Could you check a few things on this model? Use its own coordinates, in mm. A direction names the side the tool comes from. Round coordinates to 2 decimals unless told otherwise and drop trailing zeros. Write each loop counter-clockwise with the first axis right and the second up, starting at its lowest first coordinate (ties: lowest second). Pieces come first, ordered by that corner, then holes.
```python
from build123d import *

# Parameters (mm, degrees)
CROQUIS1_R              = 1.625
SALIENTE_EXTRUIR1_DEPTH = 2
SALIENTE_EXTRUIR2_START = 29.75
CROQUIS3_R              = 15
SALIENTE_EXTRUIR2_DEPTH = 29.75


with BuildPart() as part:
    # Croquis1 → Saliente-Extruir1 (new body)
    with BuildSketch(Plane.XY):
        with BuildLine():
            Line((21.447717133, -26.771381771), (20.476335362, -25.8))
            Line((20.476335362, -25.8), (21.447717133, -24.828618229))
            ThreePointArc((21.447717133, -24.828618229), (16.643597251, -14.13273811), (5.947717133, -9.328618229))
            Line((5.947717133, -9.328618229), (4.976335362, -10.3))
            Line((4.976335362, -10.3), (4.00495359, -9.328618229))
            ThreePointArc((4.00495359, -9.328618229), (-6.690926528, -14.13273811), (-11.49504641, -24.828618229))
            Line((-11.49504641, -24.828618229), (-10.523664638, -25.8))
            Line((-10.523664638, -25.8), (-11.49504641, -26.771381771))
            ThreePointArc((-11.49504641, -26.771381771), (-6.690926528, -37.46726189), (4.00495359, -42.271381771))
            Line((4.00495359, -42.271381771), (4.976335362, -41.3))
            Line((4.976335362, -41.3), (5.947717133, -42.271381771))
            ThreePointArc((5.947717133, -42.271381771), (16.643597251, -37.46726189), (21.447717133, -26.771381771))
        make_face()
        with Locations((4.976335362, -25.8)):
            Circle(CROQUIS1_R, mode=Mode.SUBTRACT)
        with Locations((-2.023664638, -25.8)):
            Circle(CROQUIS1_R, mode=Mode.SUBTRACT)
        with Locations((4.976335362, -18.8)):
            Circle(CROQUIS1_R, mode=Mode.SUBTRACT)
        with Locations((11.976335362, -25.8)):
            Circle(CROQUIS1_R, mode=Mode.SUBTRACT)
        with Locations((4.976335362, -32.8)):
            Circle(CROQUIS1_R, mode=Mode.SUBTRACT)
    extrude(amount=SALIENTE_EXTRUIR1_DEPTH)

    # Croquis3 → Saliente-Extruir2 (add)
    with BuildSketch(Plane(origin=(0, 0, 0), x_dir=(-1, 0, 0), z_dir=(0, 0, -1)).offset(SALIENTE_EXTRUIR2_START)):
        with BuildLine():
            Line((-5.947717133, -9.328618229), (-4.976335362, -10.3))
            Line((-4.976335362, -10.3), (-4.00495359, -9.328618229))
            ThreePointArc((-4.00495359, -9.328618229), (6.690926528, -14.13273811), (11.49504641, -24.828618229))
            Line((11.49504641, -24.828618229), (10.523664638, -25.8))
            Line((10.523664638, -25.8), (11.49504641, -26.771381771))
            ThreePointArc((11.49504641, -26.771381771), (6.690926528, -37.46726189), (-4.00495359, -42.271381771))
            Line((-4.00495359, -42.271381771), (-4.976335362, -41.3))
            Line((-4.976335362, -41.3), (-5.947717133, -42.271381771))
            ThreePointArc((-5.947717133, -42.271381771), (-16.643597251, -37.46726189), (-21.447717133, -26.771381771))
            Line((-21.447717133, -26.771381771), (-20.476335362, -25.8))
            Line((-20.476335362, -25.8), (-21.447717133, -24.828618229))
            ThreePointArc((-21.447717133, -24.828618229), (-16.643597251, -14.13273811), (-5.947717133, -9.328618229))
        make_face()
        with Locations((-4.976335362, -25.8)):
            Circle(CROQUIS3_R, mode=Mode.SUBTRACT)
    extrude(amount=-SALIENTE_EXTRUIR2_DEPTH)


solid = part.part
```
Q1. I'm going to push flat-ended pins straight in: pin 1 Ø8 at (y, z) = (-14, -7.5) entering from +X; pin 2 Ø3 at (x, z) = (-2.5, -16.5) entering from +Y; pin 3 Ø4 at (y, z) = (-29.5, -12) entering from +X. Where does each tip first touch, or does it pass through?
Q2. On a 3-axis mill with a long thin cutter (end or side, diameter ignored), from which of +Z, -Z, +X, -X, +Y, -Y can I reach the whole of each face in a straight line? I mean faces 5 (the flat face through (20.969, -26.292, -14.097)), 6 (the flat face through (-11.003, -26.279, -14.097)), 7 (the flat face through (5.455, -41.779, -14.097)). Say none if no direction works.
Q3. Imagine slicing it at B-B, the plane y = -18.8. Write out the boundary of the cut face in (x, z), then the cut area to 3 significant figures.
Q4. We'd pull the mould along X, two halves only. Please class faces 1 (the flat face through (5, -29, 2)), 2 (the flat face through (4.497, -9.821, -14.097)), 3 (the flat face through (5.469, -9.808, -14.097)), 4 (the cylindrical face through (-6.809, -37.348, -14.097)): pulls with the +X half, pulls with the -X half, needs draft (parallel to the pull), parting line crosses it, or undercut.
Q5. Imagine slicing it at C-C, the plane x = -2.5. Write out the boundary of the cut face in (y, z).
Q6. Imagine slicing it at D-D, the plane x = 2. Write out the boundary of the cut face in (y, z), then the cut area to 3 significant figures.
Q7. If I drill on L1, parallel to Z at x = 0, y = -38; L2, parallel to Y at x = 6, z = -1; L3, parallel to Y at x = -6.5, z = -2, over which ranges is the centre line in solid material (lowest first)?
Q8. Imagine slicing it at A-A, the plane z = -8.5. Write out the boundary of the cut face in (x, y), then the cut area to 3 significant figures.
Results found:
1. pin 1: stops at x = 19.52
1. pin 2: stops at y = -10.42
1. pin 3: stops at x = 21.39
2. face 5: +Z, -Z, +X
2. face 6: +Z, -Z, -X
2. face 7: +Z, -Z, -Y
3. outline: (-9.97, -29.75) - (-8.29, -29.75) - (-8.29, 0) - (3.35, 0) - (3.35, 2) - (-9.97, 2) - close; (6.6, 0) - (18.24, 0) - (18.24, -29.75) - (19.92, -29.75) - (19.92, 2) - (6.6, 2) - close
3. area: 153 mm2
4. face 1: needs draft
4. face 2: undercut
4. face 3: undercut
4. face 4: pulls with the -X half
5. outline: (-40.51, -29.75) - (-38.8, -29.75) - (-38.8, 0) - (-27.35, 0) - (-27.35, 2) - (-40.51, 2) - close; (-24.25, 0) - (-12.8, 0) - (-12.8, -29.75) - (-11.09, -29.75) - (-11.09, 2) - (-24.25, 2) - close
6. outline: (-42.03, -29.75) - (-40.5, -29.75) - (-40.5, 0) - (-11.1, 0) - (-11.1, -29.75) - (-9.57, -29.75) - (-9.57, 2) - (-42.03, 2) - close
6. area: 156 mm2
7. L1: z = 0 to 2
7. L2: y = -42.27 to -40.77, -10.83 to -9.33
7. L3: y = -37.66 to -35.46, -16.14 to -13.94
8. outline: (-11.5, -26.77) arc R16.5 ccw to (4, -42.27) - (4.98, -41.3) - (5.95, -42.27) arc R16.5 ccw to (21.45, -26.77) - (20.48, -25.8) - (21.45, -24.83) arc R16.5 ccw to (5.95, -9.33) - (4.98, -10.3) - (4, -9.33) arc R16.5 ccw to (-11.5, -24.83) - (-10.52, -25.8) - close; hole circle Ø30 at (4.98, -25.8)
8. area: 145 mm2
